Design review of the part shown in the three views and the two pictorial views. Dimensions are in mm from the part's minimum x, y and z. A direction names the side the tool comes from. Round coordinates to 2 decimals unless told otherwise and drop trailing zeros. Write each loop counter-clockwise with the first axis right and the second up, starting at its lowest first coordinate (ties: lowest second). Pieces come first, ordered by that corner, then holes. Notation, with made-up numbers: (-9, 11.5) -> (28, 11.5) arc R29 ccw to (28, 48.5) -> close; hole circle Ø4 at (69.25, 11.5). An arc over 180 degrees is marked (long way). Answer as a JSON object with one key per item and string values. Group by question number.
1) We need section D-D, the plane y = 3.5. Write out the cut boundary in (x, z).
2) To check wall thickness, follow probe 1 along Y at (x, z) = (10.75, 29); probe 2 along X at (y, z) = (2, 26); probe 3 along Z at (x, y) = (17.75, 13). State the ranges of each line that lie inside material, in increasing order. Write a range as [from, to].
3) Insertion check: pin 1 Ø1.5 at (x, z) = (7, 6.5) entering from -Y; pin 2 Ø1.3 at (y, z) = (2, 21) entering from +X; pin 3 Ø6 at (y, z) = (10, 13.5) entering from +X; pin 4 Ø5 at (x, y) = (4, 2.5) entering from -Z. Each pin has a flat end and moves straight along its axis. Give the tip position at first contact, or say it passes through.
4) We need section A-A, the plane x = 16.5. Write out the cut boundary in (y, z), then the cut area to 3 significant figures.
5) We need section B-B, the plane y = 18. Write out the cut boundary in (x, z), then the cut area to 3 significant figures.
6) We need section C-C, the plane z = 6.5. Write out the cut boundary in (x, y).
7) Machinability: for the marked faces 1, 2, 3, 4 and 5, which of the approach directions +Z, -Z, +X, -X, +Y, -Y give a long, thin tool a straight path to every point of the face, cutting with its end or side? Answer none if there is none.
8) Mouldability with a two-part tool opening along Z and no side actions: class the marked faces 6, 7 and 8 as pulls with the +Z half, pulls with the -Z half, needs draft (parallel to the pull), parting line crosses it, or undercut.
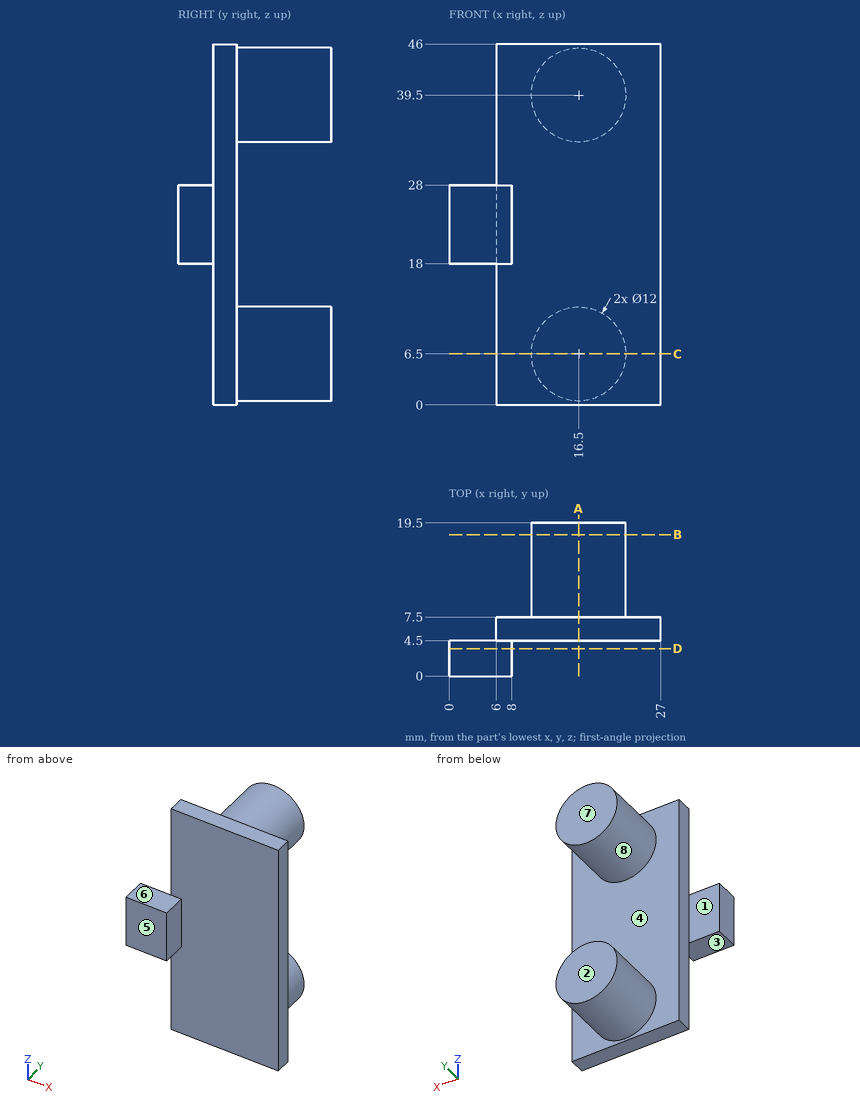
Here are the results:
{
 "1": {"outline": "(0, 18) -> (8, 18) -> (8, 28) -> (0, 28) -> close"},
 "2": {"probe 1": "y = [4.5, 7.5]", "probe 2": "x = [0, 8]", "probe 3": "z = [0.63, 12.37], [33.63, 45.37]"},
 "3": {"pin 1": "stops at y = 4.5", "pin 2": "stops at x = 8", "pin 3": "stops at x = 27", "pin 4": "stops at z = 18"},
 "4": {"outline": "(4.5, 0) -> (7.5, 0) -> (7.5, 0.5) -> (19.5, 0.5) -> (19.5, 12.5) -> (7.5, 12.5) -> (7.5, 33.5) -> (19.5, 33.5) -> (19.5, 45.5) -> (7.5, 45.5) -> (7.5, 46) -> (4.5, 46) -> close", "area": "426 mm^2"},
 "5": {"outline": "circle Ø12 at (16.5, 6.5); circle Ø12 at (16.5, 39.5)", "area": "226 mm^2"},
 "6": {"outline": "(6, 4.5) -> (27, 4.5) -> (27, 7.5) -> (22.5, 7.5) -> (22.5, 19.5) -> (10.5, 19.5) -> (10.5, 7.5) -> (6, 7.5) -> close"},
 "7": {"face 1": "+Z, -Z, -X, +Y", "face 2": "+Z, -Z, +X, -X, +Y", "face 3": "-Z, +X, -X, -Y", "face 4": "+Y", "face 5": "+Z, -Z, +X, -X, -Y"},
 "8": {"face 6": "pulls with the +Z half", "face 7": "needs draft", "face 8": "undercut"}
}
